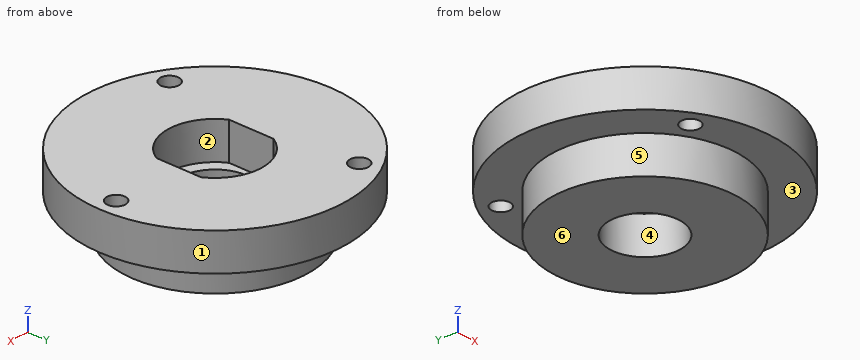
```python
from build123d import *

# Parameters (mm, degrees)
SKETCH1_R           = 7.9375
BOSS_EXTRUDE1_DEPTH = 3.188
SKETCH2_R           = 11.1125
BOSS_EXTRUDE2_DEPTH = 3.17500635
CUT_EXTRUDE2_DEPTH  = 3.17500635
CUT_EXTRUDE3_REACH  = 18.955
SKETCH4_R           = 3
CUT_EXTRUDE5_REACH  = 18.955
SKETCH5_R           = 0.79375


with BuildPart() as part:
    # Sketch1 → Boss-Extrude1 (new body)
    with BuildSketch(Plane.XY):
        Circle(SKETCH1_R)
    extrude(amount=BOSS_EXTRUDE1_DEPTH)

    # Sketch2 → Boss-Extrude2 (add)
    with BuildSketch(Plane.XY.offset(3.188)):
        Circle(SKETCH2_R)
    extrude(amount=BOSS_EXTRUDE2_DEPTH)

    # Sketch3 → Cut-Extrude2 (cut)
    with BuildSketch(Plane.XY.offset(6.36300635)):
        with BuildLine():
            Line((3.499995393, -1.9365), (3.499995393, 1.9365))
            ThreePointArc((3.499995393, 1.9365), (0, 4), (-3.499995393, 1.9365))
            Line((-3.499995393, 1.9365), (-3.499995393, -1.9365))
            ThreePointArc((-3.499995393, -1.9365), (0, -4), (3.499995393, -1.9365))
        make_face()
    extrude(amount=-CUT_EXTRUDE2_DEPTH, mode=Mode.SUBTRACT)

    # Sketch4 → Cut-Extrude3 (cut, up to next)
    with BuildSketch(Plane(origin=(0, 0, 0), x_dir=(-1, 0, 0), z_dir=(0, 0, -1)), mode=Mode.PRIVATE) as cut_extrude3_sk1:
        Circle(SKETCH4_R)
    cut_extrude3_tool1 = extrude(cut_extrude3_sk1.sketch, amount=-CUT_EXTRUDE3_REACH, mode=Mode.PRIVATE) & part.part
    add(cut_extrude3_tool1.solids().sort_by_distance((0, 0, 0))[0], mode=Mode.SUBTRACT)

    # Sketch5 → Cut-Extrude5 (cut, up to next)
    with BuildSketch(Plane.XY.offset(6.36300635), mode=Mode.PRIVATE) as cut_extrude5_sk1:
        with Locations((-4.7625, 8.248891971)):
            Circle(SKETCH5_R)
    cut_extrude5_tool1 = extrude(cut_extrude5_sk1.sketch, amount=-CUT_EXTRUDE5_REACH, mode=Mode.PRIVATE) & part.part
    # Sketch5 → Cut-Extrude5 (cut, up to next)
    with BuildSketch(Plane.XY.offset(6.36300635), mode=Mode.PRIVATE) as cut_extrude5_sk2:
        with Locations((-4.7625, -8.248891971)):
            Circle(SKETCH5_R)
    cut_extrude5_tool2 = extrude(cut_extrude5_sk2.sketch, amount=-CUT_EXTRUDE5_REACH, mode=Mode.PRIVATE) & part.part
    # Sketch5 → Cut-Extrude5 (cut, up to next)
    with BuildSketch(Plane.XY.offset(6.36300635), mode=Mode.PRIVATE) as cut_extrude5_sk3:
        with Locations((9.525, 0)):
            Circle(SKETCH5_R)
    cut_extrude5_tool3 = extrude(cut_extrude5_sk3.sketch, amount=-CUT_EXTRUDE5_REACH, mode=Mode.PRIVATE) & part.part
    add(cut_extrude5_tool1.solids().sort_by_distance((-4.7625, 8.248892, 6.363006))[0], mode=Mode.SUBTRACT)
    add(cut_extrude5_tool2.solids().sort_by_distance((-4.7625, -8.248892, 6.363006))[0], mode=Mode.SUBTRACT)
    add(cut_extrude5_tool3.solids().sort_by_distance((9.525, 0, 6.363006))[0], mode=Mode.SUBTRACT)


solid = part.part
```
Design review of the part built by this model. Coordinates are the model's own, in mm. Face numbers are marked on the shaded views. A direction names the side the tool comes from. Give positions to 0.01 mm unless a question says otherwise; leave off trailing zeros. Loops run counter-clockwise (first coordinate to the right, second up) from the corner with the lowest first, then second, coordinate; pieces in that order, holes last. Notation, with made-up numbers: M 14.25,-11 L 40.25,-11 A24 cw 40.25,22 Z; hole C 31,-21 d3. An arc over 180 degrees is marked long. Return JSON: item names as keys, results as strings. Group by question number.
Item 1: We need section C-C (x = -5). Give the boundary of the cut face in (y, z), and give its area (3 significant figures).
Item 2: Insertion check: pin 1 Ø1.5 at (y, z) = (-2.5, 4) entering from +X; pin 2 Ø1.3 at (x, y) = (-4.76, -8.25) entering from +Z; pin 3 Ø1.5 at (y, z) = (-8, 1) entering from +X; pin 4 Ø1.5 at (x, z) = (0.5, 0.5) entering from -Y. Each pin has a flat end and moves straight along its axis. Give the tip position at first contact, or say it passes through.
Item 3: We need section B-B (y = 0). Give the boundary of the cut face in (x, z).
Item 4: For probe 1 along Y at (x, z) = (0, 1.5); probe 2 along X at (y, z) = (-2, 2.5); probe 3 along X at (y, z) = (0.25, 6.25), list the stretches that pass through material, from the lowest coordinate up.
Item 5: We need section A-A (x = 0). Give the boundary of the cut face in (y, z).
Item 6: Mouldability with a two-part tool opening along X and no side actions: class the marked faces 4, 5 and 6 as released by +X, released by -X, zero draft, split by the parting line, or undercut.
Item 7: Tool access review of the marked faces 1, 2 and 3: name each direction out of +Z, -Z, +X, -X, +Y, -Y from which nothing blocks a thin tool from reaching the whole face with its end or side.
Item 8: We need section D-D (z = 6). Give the boundary of the cut face in (x, y) (1 decimal).
Output:
{
 "1": {"outline": "M -9.92,3.19 L -9.01,3.19 L -9.01,6.36 L -9.92,6.36 Z; M -7.49,3.19 L -6.16,3.19 L -6.16,0 L 6.16,0 L 6.16,3.19 L 7.49,3.19 L 7.49,6.36 L -7.49,6.36 Z; M 9.01,3.19 L 9.92,3.19 L 9.92,6.36 L 9.01,6.36 Z", "area": "92.7 mm^2"},
 "2": {"pin 1": "stops at x = 10.97", "pin 2": "passes through", "pin 3": "stops at x = 3.23", "pin 4": "stops at y = -7.94"},
 "3": {"outline": "M -11.11,3.19 L -7.94,3.19 L -7.94,0 L -3,0 L -3,3.19 L -3.5,3.19 L -3.5,6.36 L -11.11,6.36 Z; M 3,0 L 7.94,0 L 7.94,3.19 L 8.73,3.19 L 8.73,6.36 L 3.5,6.36 L 3.5,3.19 L 3,3.19 Z; M 10.32,3.19 L 11.11,3.19 L 11.11,6.36 L 10.32,6.36 Z"},
 "4": {"probe 1": "y = -7.94 to -3, 3 to 7.94", "probe 2": "x = -7.68 to -2.24, 2.24 to 7.68", "probe 3": "x = -11.11 to -3.5, 3.5 to 8.77, 10.28 to 11.11"},
 "5": {"outline": "M -11.11,3.19 L -7.94,3.19 L -7.94,0 L -3,0 L -3,3.19 L -4,3.19 L -4,6.36 L -11.11,6.36 Z; M 3,0 L 7.94,0 L 7.94,3.19 L 11.11,3.19 L 11.11,6.36 L 4,6.36 L 4,3.19 L 3,3.19 Z"},
 "6": {"face 4": "undercut", "face 5": "split by the parting line", "face 6": "zero draft"},
 "7": {"face 1": "+Z, -Z", "face 2": "+Z", "face 3": "-Z"},
 "8": {"outline": "C 0,0 d22.2; hole C -4.8,-8.2 d1.6; hole C -4.8,8.2 d1.6; hole M -3.5,-1.9 A4 ccw 3.5,-1.9 L 3.5,1.9 A4 ccw -3.5,1.9 Z; hole C 9.5,0 d1.6"}
}
